Geometry check sheet. Reference: the model listing, model coordinates, mm. Give positions to 0.01 mm unless a question says otherwise; leave off trailing zeros. Write each loop counter-clockwise with the first axis right and the second up, starting at its lowest first coordinate (ties: lowest second). Pieces come first, ordered by that corner, then holes. Notation, with made-up numbers: (24, 16) -> (29, 16) arc R22 ccw to (29, 29) -> close; hole circle Ø8 at (5, 47). An arc over 180 degrees is marked (long way). Write item = value, one per line. Start each with the question number.
1. Cross-section at B-B, the plane x = 0. Record the cut outline in (y, z).
2. Cross-section at A-A, the plane z = 0. Record the cut outline in (x, y), plus the area to 4 significant figures.
3. Mould release check, pull along Z, two halves, no side actions. Record for faces 1 (the cylindrical face through (1.05, 6.84, -0.33)), 2 (the flat face through (-1, 0, -1)), 3 (the cylindrical face through (0.867, 7.395, 3.905)): pulls with the +Z half, pulls with the -Z half, needs draft (parallel to the pull), parting line crosses it, or undercut.
4. Cross-section at C-C, the plane y = 13. Record the cut outline in (x, z), plus the area to 3 significant figures.
5. Depth check by flat-ended pin: P1, Ø1.3, axis at x = 0, z = 0, coming from the -Y side; P2, Ø1, axis at x = 3, y = 7.5, coming from the +Z side; P3, Ø4, axis at y = 12.5, z = -3, coming from the -X side. Enter the tip coordinate at first touch or a pass-through.
6. Cross-section at D-D, the plane x = -3. Record the cut outline in (y, z).
7. Thickness scan on line 1 along Z through (x, y) = (0, 3.5); line 2 along X through (y, z) = (9, 0.5); line 3 along X through (y, z) = (7.5, 1). Record the ranges inside material, lowest first.
Autodesk Inventor part; units mm, degrees
ref_plane "YZ Plane" through (0, 0, 0) normal (1, 0, 0) x (0, 1, 0)
ref_plane "XZ Plane" through (0, 0, 0) normal (0, 1, 0) x (-1, 0, 0)
ref_plane "XY Plane" through (0, 0, 0) normal (0, 0, 1) x (1, 0, 0)
sketch "Sketch1" plane through (0, 0, 0) normal (0, 1, 0) x (-1, 0, 0)
  circle A0 centre (0, 0) radius 4
  dimension "d0" = 8
extrude "Extrusion1" add sketch "Sketch1" along normal blind 15
sketch "Sketch2" plane through (0, 15, 0) normal (0, 1, 0) x (1, 0, 0)
  circle A0 centre (0, 0) radius 1.1
  dimension "d3" = 2.2
extrude "Extrusion2" cut sketch "Sketch2" against normal through all
chamfer "Chamfer1" distance 1.5 angle 45 1 edges at (-1.1, 15, 0)
properties part number "axe_bottom"
Answers:
q1.outline = (0, -4) -> (15, -4) -> (15, -2.6) -> (13.5, -1.1) -> (0, -1.1) -> close; (0, 1.1) -> (13.5, 1.1) -> (15, 2.6) -> (15, 4) -> (0, 4) -> close
q2.outline = (-4, 0) -> (-1.1, 0) -> (-1.1, 13.5) -> (-2.6, 15) -> (-4, 15) -> close; (1.1, 0) -> (4, 0) -> (4, 15) -> (2.6, 15) -> (1.1, 13.5) -> close
q2.area = 84.75 mm^2
q3.face_1 = undercut
q3.face_2 = needs draft
q3.face_3 = parting line crosses it
q4.outline = circle Ø8 at (0, 0); hole circle Ø2.2 at (0, 0)
q4.area = 46.5 mm^2
q5.P1 = through
q5.P2 = 3.12
q5.P3 = -3.87
q6.outline = (0, -2.65) -> (15, -2.65) -> (15, 2.65) -> (0, 2.65) -> close
q7.line_1 = -4 to -1.1, 1.1 to 4
q7.line_2 = -3.97 to -0.98, 0.98 to 3.97
q7.line_3 = -3.87 to -0.46, 0.46 to 3.87
